Geometry check sheet. Reference: the model listing, model coordinates, mm. Face numbers are marked on the shaded views. Round coordinates to 2 decimals unless told otherwise and drop trailing zeros. Order: outer loops, then holes, each group sorted by start corner. A loop starts at its lowest first (then second) coordinate and runs counter-clockwise, first axis right, second up.
```python
from build123d import *

# Parameters (mm, degrees)
SKETCH1_R           = 1.2065
BOSS_EXTRUDE1_DEPTH = 2.54
SKETCH2_R           = 1.651
BOSS_EXTRUDE2_DEPTH = 4.7625
SKETCH3_W           = 3.175
SKETCH3_H           = 12.7
CUT_EXTRUDE1_DEPTH  = 13.97
FILLET1_R           = 3.175


with BuildPart() as part:
    # Sketch1 → Boss-Extrude1 (new body)
    with BuildSketch(Plane(origin=(0, 0, 0), x_dir=(1, 0, 0), z_dir=(0, 1, 0))):
        Polygon((-12.7, 0), (-12.7, 31.75), (-8.001, 31.75), (-8.001, 13.97), (8.001, 13.97), (8.001, 31.75), (12.7, 31.75), (12.7, 0), align=None)
        with Locations(Location((-10.3505, 29.21, 0), (0, 0, 270))):
            Circle(SKETCH1_R, mode=Mode.SUBTRACT)
        with Locations(Location((-10.3505, 16.8275, 0), (0, 0, 270))):
            Circle(SKETCH1_R, mode=Mode.SUBTRACT)
        with Locations(Location((10.3505, 29.21, 0), (0, 0, 270))):
            Circle(SKETCH1_R, mode=Mode.SUBTRACT)
        with Locations(Location((10.3505, 16.8275, 0), (0, 0, 270))):
            Circle(SKETCH1_R, mode=Mode.SUBTRACT)
    extrude(amount=BOSS_EXTRUDE1_DEPTH)

    # Sketch2 → Boss-Extrude2 (add, symmetric)
    with BuildSketch(Plane(origin=(0, 0, 0), x_dir=(0, 0, -1), z_dir=(1, 0, 0))):
        Polygon((12.7, 2.54), (6.35, 16.51), (0, 2.54), align=None)
        with Locations(Location((6.35, 8.89, 0), (0, 0, 180))):
            Circle(SKETCH2_R, mode=Mode.SUBTRACT)
    extrude(amount=BOSS_EXTRUDE2_DEPTH, both=True)

    # Sketch3 → Cut-Extrude1 (cut)
    with BuildSketch(Plane(origin=(0, 2.54, 0), x_dir=(1, 0, 0), z_dir=(0, 1, 0))):
        with Locations((0, 6.35)):
            Rectangle(SKETCH3_W, SKETCH3_H)
    extrude(amount=CUT_EXTRUDE1_DEPTH, mode=Mode.SUBTRACT)

    # Fillet1
    fillet1_edges = [part.edges().sort_by_distance(p)[0] for p in [
        (3.175, 16.51, -6.35),
        (-3.175, 16.51, -6.35),
    ]]
    fillet(fillet1_edges, radius=FILLET1_R)


solid = part.part
```
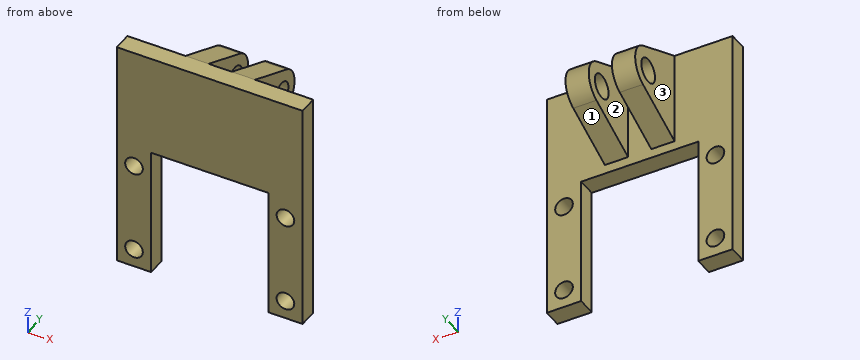
(1) Sectioned sample at B-B, the plane z = -6.35. Record the cut outline in (x, y), and give its area (3 significant figures).
Returned:
outline: (-12.7, 0) - (12.7, 0) - (12.7, 2.54) - (4.76, 2.54) - (4.76, 7.24) - (1.59, 7.24) - (1.59, 2.54) - (-1.59, 2.54) - (-1.59, 7.24) - (-4.76, 7.24) - (-4.76, 2.54) - (-12.7, 2.54) - close; (-4.76, 10.54) - (-1.59, 10.54) - (-1.59, 12.01) - (-4.76, 12.01) - close; (1.59, 10.54) - (4.76, 10.54) - (4.76, 12.01) - (1.59, 12.01) - close
area: 104 mm2
(2) Depth check by flat-ended pin: P1, Ø7.5, axis at x = 1.5, z = -16.5, coming from the +Y side; P2, Ø3, axis at y = 8.89, z = -6.35, coming from the +X side; P3, Ø5, axis at x = 1.5, y = 7, coming from the +Z side; P4, Ø2, axis at x = -5.5, y = 5, coming from the +Z side. Enter the tip coordinate at first touch or a pass-through.
Returned:
P1: stops at y = 2.54
P2: passes through
P3: stops at z = -0.89
P4: stops at z = -0.81
(3) Sectioned sample at C-C, the plane y = 9.75. Record the cut outline in (x, z), and give its area (3 significant figures).
Returned:
outline: (-4.76, -9.42) - (-1.59, -9.42) - (-1.59, -7.76) - (-4.76, -7.76) - close; (-4.76, -4.94) - (-1.59, -4.94) - (-1.59, -3.28) - (-4.76, -3.28) - close; (1.59, -9.42) - (4.76, -9.42) - (4.76, -7.76) - (1.59, -7.76) - close; (1.59, -4.94) - (4.76, -4.94) - (4.76, -3.28) - (1.59, -3.28) - close
area: 21.1 mm2
(4) Material ranges on line 1 (X direction, y = 1.35, z = -29.21); line 2 (X direction, y = 1, z = -21.5); line 3 (X direction, y = 6.5, z = -7.5), recorded low to high.
Returned:
line 1: x = -12.7 to -11.56, -9.14 to -8, 8 to 9.14, 11.56 to 12.7
line 2: x = -12.7 to -8, 8 to 12.7
line 3: x = -4.76 to -1.59, 1.59 to 4.76
(5) Sectioned sample at A-A, the plane z = -29.21. Record the cut outline in (x, y), and give its area (3 significant figures).
Returned:
outline: (-12.7, 0) - (-11.56, 0) - (-11.56, 2.54) - (-12.7, 2.54) - close; (-9.14, 0) - (-8, 0) - (-8, 2.54) - (-9.14, 2.54) - close; (8, 0) - (9.14, 0) - (9.14, 2.54) - (8, 2.54) - close; (11.56, 0) - (12.7, 0) - (12.7, 2.54) - (11.56, 2.54) - close
area: 11.6 mm2
(6) Sectioned sample at D-D, the plane x = 3.5. Record the cut outline in (y, z) (3 decimals).
Returned:
outline: (0, -13.97) - (2.54, -13.97) - (2.54, -12.7) - (10.151, -9.24) arc R3.175 ccw to (10.151, -3.46) - (2.54, 0) - (0, 0) - close; hole circle Ø3.302 at (8.89, -6.35)
(7) Draft check along X on the marked faces 1, 2 and 3. Enter one of: released by +X, released by -X, zero draft, split by the parting line, or undercut.
Returned:
face 1: zero draft
face 2: undercut
face 3: released by -X
